For this review, take the finished solid that the model builds, in its own axes (mm). A direction names the side the tool comes from. Give positions to 0.01 mm unless a question says otherwise; leave off trailing zeros. Loops run counter-clockwise (first coordinate to the right, second up) from the corner with the lowest first, then second, coordinate; pieces in that order, holes last.
```python
from build123d import *

# Parameters (mm, degrees)
SKIZZE1_R                       = 8
AUFSATZ_LINEAR_AUSTRAGEN1_DEPTH = 33.5
SKIZZE2_R                       = 3.799988553
AUFSATZ_LINEAR_AUSTRAGEN2_DEPTH = 1
VERRUNDUNG1_R                   = 1.5
VERRUNDUNG2_R                   = 0.5
SCHNITT_LINEAR_START            = -0.005
SKIZZE3_R                       = 5
SKIZZE3_R_2                     = 3.799988553
SCHNITT_LINEAR_AUSTRAGEN1_DEPTH = 0.005


with BuildPart() as part:
    # Skizze1 → Aufsatz-Linear austragen1 (new body)
    with BuildSketch(Plane(origin=(0, 0, 0), x_dir=(1, 0, 0), z_dir=(0, 1, 0))):
        with Locations(Location((0, 0, 0), (0, 0, 270))):
            Circle(SKIZZE1_R)
    extrude(amount=AUFSATZ_LINEAR_AUSTRAGEN1_DEPTH)

    # Skizze2 → Aufsatz-Linear austragen2 (add)
    with BuildSketch(Plane(origin=(0, 33.5, 0), x_dir=(1, 0, 0), z_dir=(0, 1, 0))):
        with Locations(Location((0, 0, 0), (0, 0, 270))):
            Circle(SKIZZE2_R)
    extrude(amount=AUFSATZ_LINEAR_AUSTRAGEN2_DEPTH)

    # Verrundung1
    verrundung1_edges = [part.edges().sort_by_distance(p)[0] for p in [
        (0, 0, -8),
        (0, 33.5, -8),
    ]]
    fillet(verrundung1_edges, radius=VERRUNDUNG1_R)

    # Verrundung2
    verrundung2_edges = [part.edges().sort_by_distance(p)[0] for p in [
        (0, 34.5, -3.799988553),
    ]]
    fillet(verrundung2_edges, radius=VERRUNDUNG2_R)

    # Skizze3 → Schnitt-Linear austragen1 (cut)
    with BuildSketch(Plane(origin=(0, 33.5, 0), x_dir=(1, 0, 0), z_dir=(0, 1, 0)).offset(SCHNITT_LINEAR_START)):
        with Locations(Location((0, 0, 0), (0, 0, 270))):
            Circle(SKIZZE3_R)
        with Locations(Location((0, 0, 0), (0, 0, 270))):
            Circle(SKIZZE3_R_2, mode=Mode.SUBTRACT)
    extrude(amount=SCHNITT_LINEAR_AUSTRAGEN1_DEPTH, mode=Mode.SUBTRACT)


solid = part.part
```
Item 1: Clearance check with flat-ended pins moving along their axes: pin 1 Ø1.5 at (x, y) = (-4, 17.5) entering from -Z; pin 2 Ø2 at (x, y) = (6.5, 22) entering from +Z; pin 3 Ø3 at (x, y) = (3.5, 6.5) entering from -Z. State where each tip first meets the part, or that it passes through.
Answer:
pin 1: stops at z = -7.31
pin 2: stops at z = 5.81
pin 3: stops at z = -7.75
Item 2: For L1, parallel to X at y = 33.55, z = 0; L2, parallel to Y at x = -4, z = -2.5 (3 decimals); L3, parallel to X at y = 20.5, z = -5.75, list the stretches that pass through material, from the lowest coordinate up.
Answer:
L1: x = -3.8 to 3.8
L2: y = 0 to 33.495
L3: x = -5.56 to 5.56
Item 3: Take a section at D-D on y = 32.5. Give the boundary of the cut face in (x, z).
Answer:
outline: circle Ø15.83 at (0, 0)
Item 4: Take a section at A-A on x = 0. Give the boundary of the cut face in (y, z) (3 decimals).
Answer:
outline: (0, -6.5) arc R1.5 ccw to (1.5, -8) - (32, -8) arc R1.5 ccw to (33.5, -6.5) - (33.5, -5) - (33.495, -5) - (33.495, -3.8) - (34, -3.8) arc R0.5 ccw to (34.5, -3.3) - (34.5, 3.3) arc R0.5 ccw to (34, 3.8) - (33.495, 3.8) - (33.495, 5) - (33.5, 5) - (33.5, 6.5) arc R1.5 ccw to (32, 8) - (1.5, 8) arc R1.5 ccw to (0, 6.5) - close
Item 5: Take a section at C-C on y = 28.5. Give the boundary of the cut face in (x, z), and give its area (3 significant figures).
Answer:
outline: circle Ø16 at (0, 0)
area: 201 mm2
Item 6: Tool access review of faces 1 (the flat face through (0, 0, 0)), 2 (the cylindrical face through (1.141, 33.744, 3.625)): name each direction out of +Z, -Z, +X, -X, +Y, -Y from which nothing blocks a thin tool from reaching the whole face with its end or side.
Answer:
face 1: +Z, -Z, +X, -X, -Y
face 2: +Y
Item 7: Take a section at B-B on z = 0. Give the boundary of the cut face in (x, y) (3 decimals).
Answer:
outline: (-8, 1.5) arc R1.5 ccw to (-6.5, 0) - (6.5, 0) arc R1.5 ccw to (8, 1.5) - (8, 32) arc R1.5 ccw to (6.5, 33.5) - (5, 33.5) - (5, 33.495) - (3.8, 33.495) - (3.8, 34) arc R0.5 ccw to (3.3, 34.5) - (-3.3, 34.5) arc R0.5 ccw to (-3.8, 34) - (-3.8, 33.495) - (-5, 33.495) - (-5, 33.5) - (-6.5, 33.5) arc R1.5 ccw to (-8, 32) - close
